Autodesk Inventor part; units mm, degrees
ref_plane "YZ Plane" through (0, 0, 0) normal (1, 0, 0) x (0, 1, 0)
ref_plane "XZ Plane" through (0, 0, 0) normal (0, 1, 0) x (-1, 0, 0)
ref_plane "XY Plane" through (0, 0, 0) normal (0, 0, 1) x (1, 0, 0)
sketch "Sketch1" plane through (0, 0, 0) normal (0, 0, 1) x (1, 0, 0)
  line L0 (0, 0) -> (0, 136.525)
  line L1 (-11.7886, 12.2907) -> (-39.6863, 18.4755)
  line L2 (-39.6863, 18.4755) -> (-33.3297, 47.1481)
  line L3 (-33.3297, 47.1481) -> (-5.432, 40.9633)
  line L4 (-5.432, 40.9633) -> (-11.7886, 12.2907)
  line L5 (-39.6863, 18.4755) -> (-5.432, 40.9633) construction
  line L6 (-33.3297, 47.1481) -> (-11.7886, 12.2907) construction
  circle A0 centre (-53.975, 12.7) radius 3.175
  circle A1 centre (-53.975, 12.7) radius 6.35
  line L7 (0, 0) -> (-54.712, 6.3929)
  line L8 (-59.6703, 15.5082) -> (0, 136.525)
  line L9 (-27.1302, 45.7737) -> (-37.4529, 28.5497)
  line L10 (-11.6315, 42.3377) -> (-9.5552, 22.3649)
  line L11 (-19.3809, 44.0557) -> (-25.7374, 15.3831) construction
  line L12 (0, 92.075) -> (-19.7574, 96.4551)
  line L13 (-35.3766, 8.5768) -> (-19.8779, 5.1408)
  line L14 (-19.8779, 5.1408) -> (-21.2523, -1.0586)
  line L15 (-21.2523, -1.0586) -> (-36.751, 2.3773)
  line L16 (-36.751, 2.3773) -> (-35.3766, 8.5768)
  line L17 (-35.3766, 8.5768) -> (-41.27, 4.8223)
  line L18 (-19.8779, 5.1408) -> (-17.9381, 2.096)
  line L19 (-5.432, 40.9633) -> (-33.3297, 47.1481)
  line L20 (-33.3297, 47.1481) -> (-32.2475, 52.0296)
  line L21 (-32.2475, 52.0296) -> (-4.3498, 45.8448)
  line L22 (-4.3498, 45.8448) -> (-5.432, 40.9633)
  line L23 (-53.2878, 15.7997) -> (-53.975, 12.7) construction
  line L24 (-53.975, 12.7) -> (-57.0747, 13.3872) construction
  line L25 (-27.6272, 6.8588) -> (-34.4992, -24.1386) construction
  line L26 (-31.8676, 50.076) -> (-5.5198, 44.2349)
  line L27 (-5.5198, 44.2349) -> (-4.489, 48.8845)
  line L28 (-4.489, 48.8845) -> (-30.8368, 54.7256)
  line L29 (-30.8368, 54.7256) -> (-31.8676, 50.076)
  line L30 (-31.3522, 52.4008) -> (-5.0044, 46.5597) construction
  circle A2 centre (-29.0274, 51.8854) radius 1.4732
  circle A3 centre (-22.8279, 50.5111) radius 1.4732
  circle A4 centre (-16.6284, 49.1367) radius 1.4732
  circle A5 centre (-10.4289, 47.7623) radius 1.4732
  circle A6 centre (-10.3614, 84.7398) radius 1.4732
  line L31 (-53.975, 12.7) -> (-13.3751, 95.0402)
  line L32 (-32.2923, 56.6744) -> (0, 49.5153)
  circle A7 centre (-10.3614, 84.7398) radius 4.7625
  line L33 (-4.7625, 50.5712) -> (-4.7625, 93.1308)
  line L34 (-27.5056, 55.6132) -> (-14.3936, 82.2055)
  line L35 (-5.6003, 84.6261) -> (-4.7625, 84.4403)
  circle A8 centre (-12.7, 6.35) radius 1.4224
  line L36 (-9.525, 4.7625) -> (-17.9381, 2.096)
  line L37 (-9.525, 7.9375) -> (-9.525, 4.7625)
  line L38 (-9.525, 7.9375) -> (0, 7.9375)
  line L39 (0, 13.4938) -> (-4.7625, 13.4937) construction
  line L40 (-4.7625, 13.4937) -> (-4.7625, 24.6063) construction
  line L41 (-4.7625, 24.6063) -> (0, 24.6063) construction
  line L42 (0, 24.6063) -> (0, 13.4938) construction
  line L43 (-4.7625, 19.05) -> (0, 19.05) construction
  circle A9 centre (-2.3812, 19.05) radius 1.4224
  line L44 (-4.7625, 57.15) -> (0, 57.15) construction
  circle A10 centre (-2.3813, 57.15) radius 1.4224
  circle A11 centre (-2.3813, 63.5) radius 1.4224
  circle A12 centre (-2.3813, 69.85) radius 1.4224
  circle A13 centre (-2.3813, 76.2) radius 1.4224
  line L45 (-34.4992, -24.1386) -> (-14.5705, 65.7539) construction
  line L46 (-14.5705, 65.7539) -> (-17.3193, 53.3549) construction
  line L47 (-17.3193, 53.3549) -> (-11.1198, 51.9805) construction
  line L48 (-11.1198, 51.9805) -> (-8.371, 64.3795) construction
  line L49 (-8.371, 64.3795) -> (-14.5705, 65.7539) construction
  line L50 (-14.2195, 52.6677) -> (-11.4708, 65.0667) construction
  line L51 (-15.9449, 59.5544) -> (-9.7454, 58.18) construction
  line L52 (-17.3193, 53.3549) -> (-9.7454, 58.18) construction
  line L53 (-14.5705, 65.7539) -> (-9.7454, 58.18) construction
  circle A14 centre (-13.5323, 55.7675) radius 1.4224
  circle A15 centre (-12.1579, 61.967) radius 1.4224
  line L54 (-14.2195, 52.6677) -> (-12.1579, 61.967) construction
  line L55 (-11.1198, 51.9805) -> (-9.0582, 61.2798)
  line L56 (-15.2577, 62.6542) -> (-17.3193, 53.3549)
  arc A16 (-17.3193, 53.3549) -> (-11.1198, 51.9805) centre (-14.2195, 52.6677) ccw construction
  arc A17 (-9.0582, 61.2798) -> (-15.2577, 62.6542) centre (-12.1579, 61.967) ccw
  point P0 (-22.5591, 29.7194)
  point P1 (-20.4869, 2.3938)
  point P2 (-36.3367, 4.2458)
  point P3 (-51.1668, 18.3953)
  point P4 (-4.7625, 7.9375)
  point P5 (-22.5591, 29.7194)
  point P6 (-13.1887, 57.3173)
  dimension "d13" = 136.525
  dimension "d14" = 29.3687
  dimension "d15" = 28.575
  dimension "d16" = 12.5
  dimension "d17" = 6.35
  dimension "d19" = 53.975
  dimension "d22" = 12.7
  dimension "d23" = 7.9375
  dimension "d24" = 19.05
  dimension "d26" = 102.5
  dimension "d29" = 6.35
  dimension "d31" = 7.9375
  dimension "d34" = 5
  dimension "d35" = 26.9875
  dimension "d38" = 31.75
  dimension "d40" = 26.9875
  dimension "d41" = 4.7625
  dimension "d42" = 2.9464
  dimension "d43" = 2.3813
  dimension "d46" = 6.35
  dimension "d51" = 2.9464
  dimension "d52" = 79.7719
  dimension "d53" = 6.35
  dimension "d54" = 9.525
  dimension "d55" = 4.7625
  dimension "d56" = 4.7625
  dimension "d60" = 12.7
  dimension "d61" = 3.175
  dimension "d66" = 2.8448
  dimension "d67" = 12.7
  dimension "d72" = 8.7312
  dimension "d75" = 34.925
  dimension "d80" = 92.075
  dimension "d81" = 6.35
  dimension "d82" = 7.9375
  dimension "d83" = 3.175
  dimension "d84" = 9.525
  dimension "d85" = 4.7625
  dimension "d86" = 11.1125
  dimension "d87" = 2.8448
  dimension "d88" = 19.05
  dimension "d89" = 2.8448
  dimension "d90" = 38.1
  dimension "d93" = 6.35
  dimension "d98" = 92.075
  dimension "d99" = 12.7
  dimension "d100" = 6.35
  dimension "d101" = 2.8448
  dimension "d102" = 2.8448
extrude "Extrusion1" add sketch "Sketch1" along normal blind 6.35 contours L38 L37 L36 L18 L13 L17 L7 A1 L31 L32 L0 | L32 L33 L12 L0 | L33 L35 A7 L34 L32 L31 L12 | A7 | A1 | L3 L20 L21 L29 L26 L27 L22 | L27 L26 L29 L21 A2 A3 A4 A5 | L21 A5 A4 A3 A2 L29 L28 L27
fillet "Fillet1" radius 2.3813 17 edges at (-39.6863, 18.4755, 3.175) (-11.7886, 12.2907, 3.175) (-51.1668, 18.3953, 3.175) (-19.8779, 5.1408, 3.175) (-35.3766, 8.5768, 3.175) (-41.27, 4.8223, 3.175) (-13.3751, 95.0402, 3.175) (-14.3936, 82.2055, 3.175) (-5.6003, 84.6261, 3.175) (-4.7625, 84.4403, 3.175) (-27.5056, 55.6132, 3.175) (-4.7625, 50.5712, 3.175) (-33.3297, 47.1481, 3.175) (-5.432, 40.9633, 3.175) (-17.9381, 2.096, 3.175) (-9.525, 7.9375, 3.175) (-9.525, 4.7625, 3.175)
equation "\"d56\" = d55"
properties part number "Uprights" material "Aluminum 6061"
Input: part model. Units: mm. Frame: model coordinates. A direction names the side the tool comes from. Coordinates: 2 decimals unless noted, no trailing zeros. Write each loop counter-clockwise with the first axis right and the second up, starting at its lowest first coordinate (ties: lowest second). Pieces come first, ordered by that corner, then holes. Notation, with made-up numbers: (-34.75, 39) -> (-15.75, 39) arc R20 cw to (-15.75, 43) -> close; hole circle Ø5 at (-4.75, -5.5). An arc over 180 degrees is marked (long way). Answer as a JSON object with one key per item and string values.
1. Mould query, pull axis X, two halves, no side actions, for faces 3 (the face through (-48.324, 5.646, 3.131)), 4 (the face through (-2.57, 55.74, 3.13)), 5 (the face through (-2.57, 68.44, 3.13)), 6 (the face through (-4, 7.938, 3)). Classes: released by +X, released by -X, zero draft, split by the parting line, or undercut.
Result set:
{"face 3": "released by -X", "face 4": "undercut", "face 5": "undercut", "face 6": "zero draft"}
2. Access query for faces 1 (the face through (-5.63, 51.7, 3.13)), 2 (the face through (-38.352, 6.682, 3.131)). Directions: +Z, -Z, +X, -X, +Y, -Y. A direction counts if a zero-diameter tool reaches every point of the face in a straight line with its end or side. Return the directions, or none.
Result set:
{"face 1": "+Z, -Z", "face 2": "+Z, -Z, -Y"}
3. Section A-A on y = 69.85. Return the cut outline in (x, z).
Result set:
{"outline": "(-25.8, 0) -> (-20.49, 0) -> (-20.49, 6.35) -> (-25.8, 6.35) -> close; (-4.76, 0) -> (-3.8, 0) -> (-3.8, 6.35) -> (-4.76, 6.35) -> close; (-0.96, 0) -> (0, 0) -> (0, 6.35) -> (-0.96, 6.35) -> close"}
4. Section D-D on z = 4.5. Count the separate pieces of the cut face and the enclosed holes in it, then the cut area to 3 significant figures.
Result set:
{"separate pieces": "1", "enclosed holes": "14", "area": "1,780 mm2"}
5. First-contact query: P1, Ø3, axis at y = 69, z = 4.5, coming from the -X side; P2, Ø1.9, axis at x = -3, z = 2.5, coming from the -Y side; P3, Ø1.5, axis at y = 73, z = 5, coming from the -X side. Flat tips, straight axial feed; report the tip coordinate or a pass-through.
Result set:
{"P1": "stops at x = -26.95", "P2": "stops at y = 7.94", "P3": "stops at x = -24.61"}
6. Section C-C on x = -43. Return the cut outline in (y, z), then the cut area to 3 significant figures.
Result set:
{"outline": "(5.02, 0) -> (34.96, 0) -> (34.96, 6.35) -> (5.02, 6.35) -> close", "area": "190 mm2"}
7. Section B-B on y = 57.15. Return the cut outline in (x, z), then the cut area to 3 significant figures.
Result set:
{"outline": "(-32.06, 0) -> (-26.41, 0) -> (-26.41, 6.35) -> (-32.06, 6.35) -> close; (-4.76, 0) -> (-3.8, 0) -> (-3.8, 6.35) -> (-4.76, 6.35) -> close; (-0.96, 0) -> (0, 0) -> (0, 6.35) -> (-0.96, 6.35) -> close", "area": "48.1 mm2"}
8. Material intervals for line 1 (Y direction, x = -3, z = 1); line 2 (Y direction, x = -17, z = 0.5); line 3 (Y direction, x = -21.5, z = 5.5), sorted ascending. Write a range as from..to.
Result set:
{"line 1": "y = 7.94..17.77, 20.33..55.87, 58.43..62.22, 64.78..68.57, 71.13..74.92, 77.48..92.74", "line 2": "y = 2.54..13.45, 43.53..47.71, 50.56..53.28, 76.92..87.69", "line 3": "y = 5.5..14.44, 44.53..49.87, 51.15..54.28, 67.79..78.56"}
